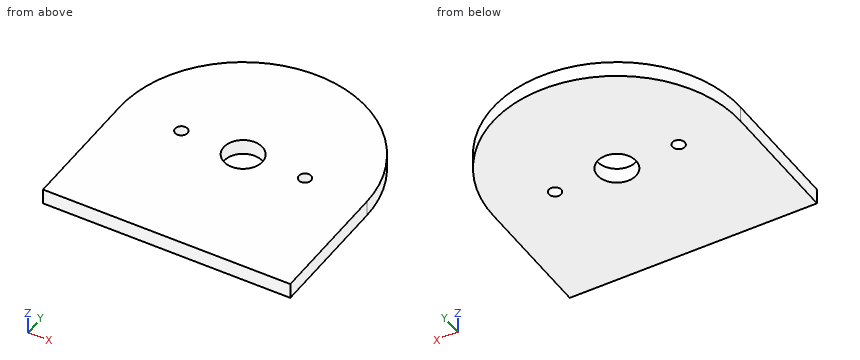
Autodesk Inventor part; units mm, degrees
sketch "Sketch1" plane through (0, 0, 0) normal (0, 0, 1) x (1, 0, 0)
  arc A0 (50.8, 0) -> (-50.8, 0) centre (0, 0) ccw
  line L0 (50.8, 0) -> (50.8, -52.7558)
  line L1 (50.8, -52.7558) -> (-50.8, -52.7558)
  line L2 (-50.8, -52.7558) -> (-50.8, 0)
  line L3 (0, 71.5112) -> (0, -73.467)
  dimension "d2" = 52.7558
  dimension "d3" = 50.8
  dimension "d22" = 0
extrude "Extrusion1" add sketch "Sketch1" along normal mid plane 6.35
sketch "Sketch2" plane through (0, 0, 3.175) normal (0, 0, 1) x (1, 0, 0)
  point P0 (0, 0)
  point P1 (0, 0)
hole "Hole1" at (0, 0, 3.175) direction (0, 0, -1) diameter 15.875 end through all
sketch "Sketch5" plane through (0, 0, 3.175) normal (0, 0, 1) x (1, 0, 0)
  circle A0 centre (-25.4, 0) radius 2.54
  line L0 (0, 50.8056) -> (0, 0) construction
  circle A1 centre (25.4, 0) radius 2.54
  dimension "d31" = 5.08
  dimension "d32" = 25.4
hole "Hole4" at (-25.4, 0, 3.175) at (25.4, 0, 3.175) direction (0, 0, -1) diameter 5.08 end through all
properties part number "Boom Hinge" material "Aluminum 6061"
Geometry: final body of the model. Coordinates: model frame, mm. Coordinates: 2 decimals unless noted, no trailing zeros. Order: outer loops, then holes, each group sorted by start corner. A loop starts at its lowest first (then second) coordinate and runs counter-clockwise, first axis right, second up.
(1) Material intervals for probe 1 along X at (y, z) = (0, -0.5); probe 2 along Y at (x, z) = (-25.4, 1.25); probe 3 along Y at (x, z) = (-46, -0.5), sorted ascending.
(2) Section query A-A (x = 0). Return the cut outline in (y, z) (1 decimal).
(3) Section query B-B (x = -14). Return the cut outline in (y, z) (3 decimals).
(4) Section query C-C (x = -25.4). Return the cut outline in (y, z) (3 decimals).
(5) Section query D-D (y = 35). Return the cut outline in (x, z) (3 decimals), plus the area to 3 significant figures.
Solution:
1. probe 1: x = -50.8 to -27.94, -22.86 to -7.94, 7.94 to 22.86, 27.94 to 50.8
1. probe 2: y = -52.76 to -2.54, 2.54 to 43.99
1. probe 3: y = -52.76 to 21.56
2. outline: (-52.8, -3.2) - (-7.9, -3.2) - (-7.9, 3.2) - (-52.8, 3.2) - close; (7.9, -3.2) - (50.8, -3.2) - (50.8, 3.2) - (7.9, 3.2) - close
3. outline: (-52.756, -3.175) - (48.833, -3.175) - (48.833, 3.175) - (-52.756, 3.175) - close
4. outline: (-52.756, -3.175) - (-2.54, -3.175) - (-2.54, 3.175) - (-52.756, 3.175) - close; (2.54, -3.175) - (43.994, -3.175) - (43.994, 3.175) - (2.54, 3.175) - close
5. outline: (-36.819, -3.175) - (36.819, -3.175) - (36.819, 3.175) - (-36.819, 3.175) - close
5. area: 468 mm2
